Work out the finished part from the listing and answer in its coordinate system (mm). A direction names the side the tool comes from. Give positions to 0.01 mm unless a question says otherwise; leave off trailing zeros. Loops run counter-clockwise (first coordinate to the right, second up) from the corner with the lowest first, then second, coordinate; pieces in that order, holes last. Notation, with made-up numbers: (80, 37.25) - (110, 37.25) arc R26 cw to (110, 68.25) - close; hole circle Ø1 at (16, 72.5). An arc over 180 degrees is marked (long way). One line per item, written item: value.
from build123d import *

# Parameters (mm, degrees)
F0_W     = 25
F0_H     = 90
F1_DEPTH = 2
F2_W     = 25
F2_H     = 2
F3_DEPTH = 20
F4_R     = 2
F5_DEPTH = 25
F6_R     = 3.1
F7_DEPTH = 25


with BuildPart() as f1:
    # F0 (on Front) → F1 (new body)
    with BuildSketch(Plane.XZ):
        Rectangle(F0_W, F0_H)
    extrude(amount=F1_DEPTH)

    # F2 (on face) → F3 (join)
    with BuildSketch(Plane.XZ.offset(2)):
        with Locations((0, -44)):
            Rectangle(F2_W, F2_H)
    extrude(amount=-F3_DEPTH)

    # F4 (on face) → F5 (cut)
    with BuildSketch(Plane.XZ.offset(2)):
        with Locations((7.5, 25)):
            Circle(F4_R)
        with Locations((-6.5, -3)):
            Circle(F4_R)
    extrude(amount=-F5_DEPTH, mode=Mode.SUBTRACT)

    # F6 (on face) → F7 (cut)
    with BuildSketch(Plane.XY.offset(-43)):
        with Locations((7.5, 9)):
            Circle(F6_R)
        with Locations((-7.5, 9)):
            Circle(F6_R)
    extrude(amount=-F7_DEPTH, mode=Mode.SUBTRACT)


solid = f1.part
1. Flat-ended cylindrical pins translate along their axes: pin 1 Ø8 at (x, y) = (-7.5, 9) entering from +Z; pin 2 Ø3 at (x, z) = (9, 4) entering from +Y; pin 3 Ø2.5 at (x, z) = (7.5, 25) entering from -Y. Find the tip coordinate at first contact, or state that the pin passes through.
Output:
pin 1: stops at z = -43
pin 2: stops at y = 0
pin 3: passes through
2. The mould has two halves that part along X. Classify faces 3 (the flat face through (0, -1, 45)), 4 (the flat face through (-12.5, -0.2, -10.2)), 5 (the cylindrical face through (-10.6, 9.1, -44)), 6 (the flat face through (12.5, -0.2, -10.2)): released by +X, released by -X, zero draft, split by the parting line, or undercut.
Output:
face 3: zero draft
face 4: released by -X
face 5: undercut
face 6: released by +X
3. Section B-B (x = 7.5) is taken. Write down the section's boundary in (y, z), and give its area (3 significant figures).
Output:
outline: (-2, -45) - (5.9, -45) - (5.9, -43) - (0, -43) - (0, 23) - (-2, 23) - close; (-2, 27) - (0, 27) - (0, 45) - (-2, 45) - close; (12.1, -45) - (18, -45) - (18, -43) - (12.1, -43) - close
area: 196 mm²
4. Find the intervals of material crossed by line 1 along Y through (x, z) = (7.5, -43.9); line 2 along Z through (x, y) = (7.5, -0.9); line 3 along Z through (x, y) = (-5.5, 11.75), in increasing order.
Output:
line 1: y = -2 to 5.9, 12.1 to 18
line 2: z = -45 to 23, 27 to 45
line 3: z = -45 to -43
5. Section A-A (y = 9) is taken. Write down the section's boundary in (x, z), and give its area (3 significant figures).
Output:
outline: (-12.5, -45) - (-10.6, -45) - (-10.6, -43) - (-12.5, -43) - close; (-4.4, -45) - (4.4, -45) - (4.4, -43) - (-4.4, -43) - close; (10.6, -45) - (12.5, -45) - (12.5, -43) - (10.6, -43) - close
area: 25.2 mm²
6. Section C-C (z = 25) is taken. Write down the section's boundary in (x, y).
Output:
outline: (-12.5, -2) - (5.5, -2) - (5.5, 0) - (-12.5, 0) - close; (9.5, -2) - (12.5, -2) - (12.5, 0) - (9.5, 0) - close
7. For faces 1 (the flat face through (0, 9, -43)), 2 (the flat face through (0, 18, -44)), determine the directions among +Z, -Z, +X, -X, +Y, -Y from which every point of the face is accessible in a straight line to the end or side of a thin tool.
Output:
face 1: +Z, +X, -X, +Y
face 2: +Z, -Z, +X, -X, +Y
8. Section D-D (x = -2) is taken. Write down the section's boundary in (y, z).
Output:
outline: (-2, -45) - (18, -45) - (18, -43) - (0, -43) - (0, 45) - (-2, 45) - close
